Could you check a few things on this drawing? It's one solid part, dimensions in mm from its lowest x, y, z. A direction names the side the tool comes from. Round coordinates to 2 decimals unless told otherwise and drop trailing zeros. Loops run counter-clockwise (first coordinate to the right, second up) from the corner with the lowest first, then second, coordinate; pieces in that order, holes last. Notation, with made-up numbers: M 21,52 L 37,52 A19 cw 37,68 Z; hole C 40.5,86.5 d3. An arc over 180 degrees is marked long. Return JSON: item names as keys, results as strings.
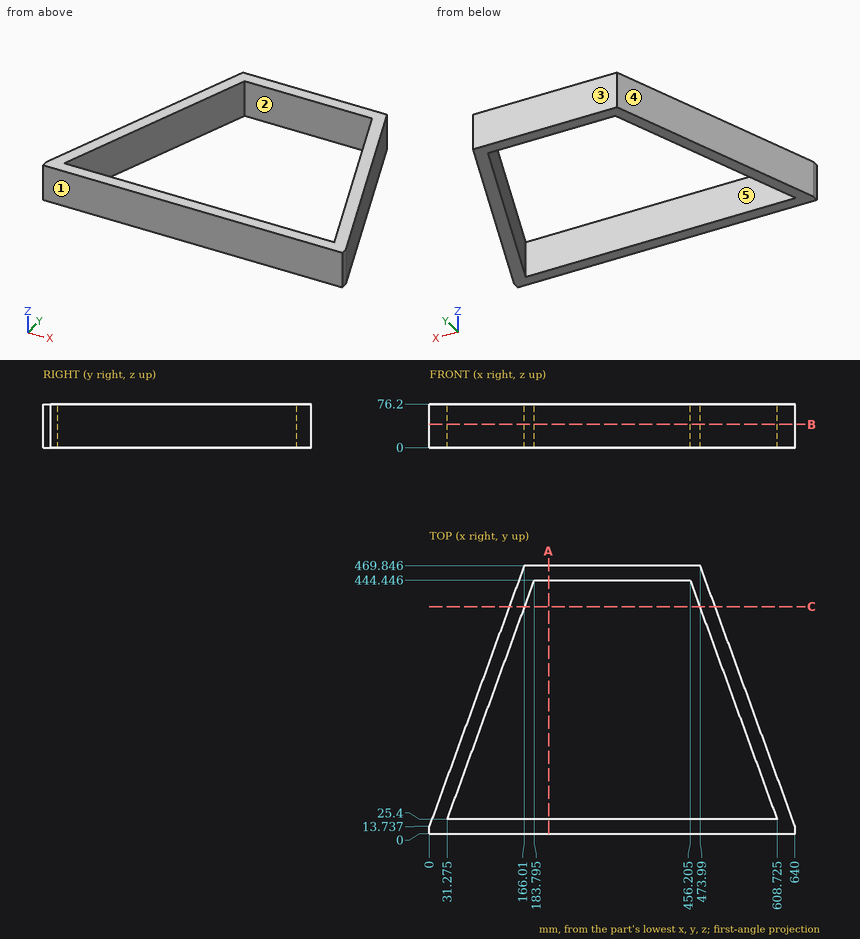
Q1. If I drill on line 1 along Y through (x, z) = (209.5, 10.5); line 2 along X through (y, z) = (303.5, 73.5) (1 decimal); line 3 along X through (y, z) = (129, 34), over which ranges is the centre line in solid material (lowest first)?
Results:
{"line 1": "y = 0 to 25.4, 444.45 to 469.85", "line 2": "x = 105.5 to 132.5, 507.5 to 534.5", "line 3": "x = 41.95 to 68.98, 571.02 to 598.05"}
Q2. Suppose I cut it at B-B, the plane z = 40.5. Please give me the cut outline in (x, y) (1 decimal), plus the area to 3 significant figures.
Results:
{"outline": "M 0,0 L 640,0 L 640,13.7 L 474,469.8 L 166,469.8 L 0,13.7 Z; hole M 31.3,25.4 L 608.7,25.4 L 456.2,444.4 L 183.8,444.4 Z", "area": "46,900 mm2"}
Q3. Thinking about a two-plate mould opening in Y: for the marked faces 1, 2 and 3, which applies, pulls with the +Y half, pulls with the -Y half, needs draft (parallel to the pull), parting line crosses it, or undercut?
Results:
{"face 1": "pulls with the -Y half", "face 2": "undercut", "face 3": "pulls with the +Y half"}
Q4. Suppose I cut it at C-C, the plane y = 398. Please give me the cut outline in (x, z).
Results:
{"outline": "M 139.86,0 L 166.89,0 L 166.89,76.2 L 139.86,76.2 Z; M 473.11,0 L 500.14,0 L 500.14,76.2 L 473.11,76.2 Z"}
Q5. Suppose I cut it at A-A, the plane x = 208.5. Please give me the cut outline in (y, z), plus the area to 3 significant figures.
Results:
{"outline": "M 0,0 L 25.4,0 L 25.4,76.2 L 0,76.2 Z; M 444.45,0 L 469.85,0 L 469.85,76.2 L 444.45,76.2 Z", "area": "3,870 mm2"}
Q6. On a 3-axis mill with a long thin cutter (end or side, diameter ignored), from which of +Z, -Z, +X, -X, +Y, -Y can I reach the whole of each face in a straight line? I mean the marked faces 4 and 5. Say none if no direction works.
Results:
{"face 4": "+Z, -Z, -X, +Y", "face 5": "+Z, -Z"}
Q7. I'm going to push flat-ended pins straight in: pin 1 Ø3 at (y, z) = (158, 61) entering from +X; pin 2 Ø8 at (y, z) = (401.5, 29.5) entering from -X; pin 3 Ø3 at (y, z) = (183.5, 12) entering from +X. Where does each tip first touch, or does it pass through?
Results:
{"pin 1": "stops at x = 588.04", "pin 2": "stops at x = 139.68", "pin 3": "stops at x = 578.76"}
